```python
from build123d import *

# Parameters (mm, degrees)
DODANIE_WYCI_GNI_CIE1_DEPTH = 14.5
OTW_R_12_0_12_1_D           = 12
DODANIE_WYCI_GNI_CIE2_DEPTH = 3
DODANIE_WYCI_GNI_CIE3_START = 3
DODANIE_WYCI_GNI_CIE3_DEPTH = 3


with BuildPart() as part:
    # Szkic1 → Dodanie-wyciągnięcie1 (new, symmetric)
    with BuildSketch(Plane.XY):
        with BuildLine():
            Line((-85, 30.5), (-83, 32.5))
            Line((-83, 32.5), (-57.046389972, 32.5))
            ThreePointArc((-57.046389972, 32.5), (-56.394946898, 32.672548578), (-55.914331752, 33.144946896))
            ThreePointArc((-55.914331752, 33.144946896), (0, 65), (55.914331752, 33.144946896))
            ThreePointArc((55.914331752, 33.144946896), (56.394946898, 32.672548578), (57.046389972, 32.5))
            Line((57.046389972, 32.5), (83, 32.5))
            Line((83, 32.5), (85, 30.5))
            Line((85, 30.5), (85, 0))
            Line((85, 0), (60, 0))
            ThreePointArc((60, 0), (0, 60), (-60, 0))
            Line((-60, 0), (-85, 0))
            Line((-85, 0), (-85, 30.5))
        make_face()
    extrude(amount=DODANIE_WYCI_GNI_CIE1_DEPTH, both=True)

    # Otwór Ø12.0 (12)1 (through all)
    with Locations(Plane(origin=(0, 0, 0), x_dir=(-1, 0, 0), z_dir=(0, -1, 0))):
        with Locations((70, 0), (-70, 0)):
            Hole(OTW_R_12_0_12_1_D / 2)

    # Szkic4 → Dodanie-wyciągnięcie2 (add)
    with BuildSketch(Plane(origin=(0, 0, -14.5), x_dir=(-1, 0, 0), z_dir=(0, 0, -1))):
        with BuildLine():
            Line((-53, 0), (-85, 0))
            Line((-85, 0), (-85, 30.5))
            Line((-85, 30.5), (-83, 32.5))
            Line((-83, 32.5), (-57.046389972, 32.5))
            ThreePointArc((-57.046389972, 32.5), (-56.394946898, 32.672548578), (-55.914331752, 33.144946896))
            ThreePointArc((-55.914331752, 33.144946896), (0, 65), (55.914331752, 33.144946896))
            ThreePointArc((55.914331752, 33.144946896), (56.394946898, 32.672548578), (57.046389972, 32.5))
            Line((57.046389972, 32.5), (83, 32.5))
            Line((83, 32.5), (85, 30.5))
            Line((85, 30.5), (85, 0))
            Line((85, 0), (53, 0))
            ThreePointArc((53, 0), (0, 53), (-53, 0))
        make_face()
    extrude(amount=DODANIE_WYCI_GNI_CIE2_DEPTH)

    # Szkic5 → Dodanie-wyciągnięcie3 (add)
    with BuildSketch(Plane.XY.offset(14.5).offset(DODANIE_WYCI_GNI_CIE3_START)):
        with BuildLine():
            Line((-53, 0), (-85, 0))
            Line((-85, 0), (-85, 30.5))
            Line((-85, 30.5), (-83, 32.5))
            Line((-83, 32.5), (-57.046389972, 32.5))
            ThreePointArc((-57.046389972, 32.5), (-56.394946898, 32.672548578), (-55.914331752, 33.144946896))
            ThreePointArc((-55.914331752, 33.144946896), (0, 65), (55.914331752, 33.144946896))
            ThreePointArc((55.914331752, 33.144946896), (56.394946898, 32.672548578), (57.046389972, 32.5))
            Line((57.046389972, 32.5), (83, 32.5))
            Line((83, 32.5), (85, 30.5))
            Line((85, 30.5), (85, 0))
            Line((85, 0), (53, 0))
            ThreePointArc((53, 0), (0, 53), (-53, 0))
        make_face()
    extrude(amount=-DODANIE_WYCI_GNI_CIE3_DEPTH)


solid = part.part
```
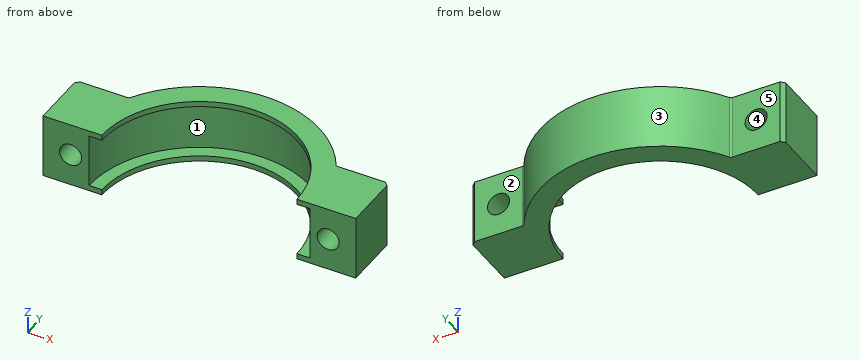
Geometry check sheet. Reference: the model listing, model coordinates, mm. Face numbers are marked on the shaded views. A direction names the side the tool comes from. Round coordinates to 2 decimals unless told otherwise and drop trailing zeros. Order: outer loops, then holes, each group sorted by start corner. A loop starts at its lowest first (then second) coordinate and runs counter-clockwise, first axis right, second up. Notation, with made-up numbers: M -15,-14.75 L 19,-14.75 A13 ccw 19,1.25 Z; hole C -39,-18.5 d8. An arc over 180 degrees is marked long. Answer as CSV lines item,"result".
1) Sectioned sample at B-B on y = 11. Record the cut outline in (x, z).
Entries:
outline,"M -85,-17.5 L -51.85,-17.5 L -51.85,-14.5 L -58.98,-14.5 L -58.98,14.5 L -51.85,14.5 L -51.85,17.5 L -85,17.5 Z; M 51.85,-17.5 L 85,-17.5 L 85,17.5 L 51.85,17.5 L 51.85,14.5 L 58.98,14.5 L 58.98,-14.5 L 51.85,-14.5 Z; hole C -70,0 d12; hole C 70,0 d12"
2) Tool access check on the marked faces 4 and 5. Record the directions out of +Z, -Z, +X, -X, +Y, -Y that give a thin tool (end or side, any length) a straight path to the whole face; none if there is none.
Entries:
face 4,"+Y, -Y"
face 5,"+Z, -Z, -X, +Y"
3) Sectioned sample at C-C on z = 0. Record the cut outline in (x, y), and give its area (3 significant figures).
Entries:
outline,"M -85,0 L -76,0 L -76,32.5 L -83,32.5 L -85,30.5 Z; M -64,0 L -60,0 A60 cw 60,0 L 64,0 L 64,32.5 L 57.05,32.5 A1.32 cw 55.91,33.14 A65 ccw -55.91,33.14 A1.32 cw -57.05,32.5 L -64,32.5 Z; M 76,0 L 85,0 L 85,30.5 L 83,32.5 L 76,32.5 Z"
area,"1,680 mm2"
4) Mould release check, pull along X, two halves, no side actions. Record for the marked faces 1, 2 and 3: +X half, -X half, draft (parallel to the pull), parting line (faces both ways), or undercut.
Entries:
face 1,"undercut"
face 2,"draft"
face 3,"parting line"
5) Gauge pin test, flat ends, axial feed: pin 1 Ø8 at (x, z) = (-71.5, 1) entering from +Y; pin 2 Ø19 at (x, z) = (-70, 0) entering from +Y; pin 3 Ø3 at (x, z) = (-45.5, 1.5) entering from +Y; pin 4 Ø12 at (x, z) = (-19.5, -11) entering from +Y. Record the tip position at first contact, or that the pin passes through.
Entries:
pin 1,"through"
pin 2,"y = 32.5"
pin 3,"y = 47.84"
pin 4,"y = 63.58"
6) Sectioned sample at A-A on x = -70. Record the cut outline in (y, z), and give its area (4 significant figures).
Entries:
outline,"M 0,-17.5 L 32.5,-17.5 L 32.5,-6 L 0,-6 Z; M 0,6 L 32.5,6 L 32.5,17.5 L 0,17.5 Z"
area,"747.5 mm2"
7) Sectioned sample at D-D on x = 0. Record the cut outline in (y, z), and give its area (3 significant figures).
Entries:
outline,"M 53,-17.5 L 65,-17.5 L 65,17.5 L 53,17.5 L 53,14.5 L 60,14.5 L 60,-14.5 L 53,-14.5 Z"
area,"217 mm2"
8) Thickness scan on probe 1 along Z at (x, y) = (70, 16.5); probe 2 along X at (y, z) = (4.5, 3); probe 3 along X at (y, z) = (16.5, 2). Record the ranges inside material, lowest first. Write a range as [from, to].
Entries:
probe 1,"[-17.5, -6], [6, 17.5]"
probe 2,"[-85, -75.2], [-64.8, -59.83], [59.83, 64.8], [75.2, 85]"
probe 3,"[-85, -75.66], [-64.34, -57.69], [57.69, 64.34], [75.66, 85]"
